For this review, take the finished solid that the model builds, in its own axes (mm). A direction names the side the tool comes from. Round coordinates to 2 decimals unless told otherwise and drop trailing zeros. Write each loop counter-clockwise with the first axis right and the second up, starting at its lowest first coordinate (ties: lowest second). Pieces come first, ordered by that corner, then holes. Notation, with made-up numbers: M 69,62.25 L 126,62.25 A19 cw 126,96.25 Z; hole C 50,52 d6. An arc over 180 degrees is marked long. Use one line per item in the form item = value. Start each with the question number.
Item 1: For faces 1 (the cylindrical face through (250.72, 2.12, 126.67)), 2 (the flat face through (284.2, 3.6, -11.4)), 3 (the cylindrical face through (270.393, 3.648, 1.982)), list the 3-axis set-ups (+Z, -Z, +X, -X, +Y, -Y) from which the entire face can be reached by the end or side of a thin tool; tool diameter is ignored.
Item 2: For line 1 (X direction, y = 1.25, z = 0.5); line 2 (Y direction, x = 275.5, z = -28); line 3 (X direction, y = 3.25, z = -28.5), list the stretches that pass through material, from the lowest coordinate up. Write a range as [from, to].
Item 3: Add section A-A (z = 92.5). State the section outline as (x, y) points.
Item 4: For P1, Ø14, axis at x = 256, z = 125, coming from the +Y side; P2, Ø1.5, axis at x = 258, z = 107, coming from the +Y side; P3, Ø3, axis at x = 257, y = 2.5, coming from the -Z side, all flat-tipped, find the tip position at first contact; note any pin that passes through.
Item 5: Draft analysis for pull direction Z (two halves, no side actions). For faces 4 (the cylindrical face through (289.992, 1.775, 2.126)), 5 (the flat face through (272, 0, 10)), 6 (the cylindrical face through (281.795, 2.121, 36.119)), state which applies: released by +Z, released by -Z, zero draft, split by the parting line, or undercut.
Item 6: Add section B-B (y = 4.75). State the section outline as (x, z) points.
Item 7: Add section C-C (z = -117). State the section outline as (x, y) points.
from build123d import *

# Parameters (mm, degrees)
AUFSATZ_LINEAR_AUSTRAGEN1_DEPTH = 3.6
SCHNITT_LINEAR_AUSTRAGEN1_DEPTH = 3
SCHNITT_LINEAR_AUSTRAGEN2_DEPTH = 325.249841943
SCHNITT_LINEAR_AUSTRAGEN3_DEPTH = 3
AUFSATZ_LINEAR_AUSTRAGEN2_DEPTH = 3.8


with BuildPart() as part:
    # Skizze1 → Aufsatz-Linear austragen1 (new body)
    with BuildSketch(Plane(origin=(0, 0, 0), x_dir=(1, 0, 0), z_dir=(0, 1, 0))):
        with BuildLine():
            Line((251.147367097, 145), (234.173269183, 135.2))
            ThreePointArc((234.173269183, 135.2), (270.4, 0), (234.173269183, -135.2))
            Line((234.173269183, -135.2), (251.147367097, -145))
            ThreePointArc((251.147367097, -145), (290, 0), (251.147367097, 145))
        make_face()
    extrude(amount=AUFSATZ_LINEAR_AUSTRAGEN1_DEPTH)

    # Skizze2 → Schnitt-Linear austragen1 (cut)
    with BuildSketch(Plane(origin=(0, 3.6, 0), x_dir=(1, 0, 0), z_dir=(0, 1, 0))):
        with BuildLine():
            Line((243.266535923, 140.45), (246.037817215, 142.05))
            ThreePointArc((246.037817215, 142.05), (284.1, 0), (246.037817215, -142.05))
            Line((246.037817215, -142.05), (243.266535923, -140.45))
            ThreePointArc((243.266535923, -140.45), (280.9, 0), (243.266535923, 140.45))
        make_face()
    extrude(amount=-SCHNITT_LINEAR_AUSTRAGEN1_DEPTH, mode=Mode.SUBTRACT)

    # Skizze3 → Schnitt-Linear austragen2 (cut, through all)
    with BuildSketch(Plane(origin=(0, 3.6, 0), x_dir=(1, 0, 0), z_dir=(0, 1, 0))):
        Polygon((276.456207793, 41.439295032), (282.404876961, 42.222452186), (283.710138883, 32.308003572), (277.761469715, 31.524846419), align=None)
        Polygon((256.310912175, -111.579417009), (261.85418937, -113.875517603), (265.681023694, -104.636722278), (260.137746499, -102.340621683), align=None)
    extrude(amount=-SCHNITT_LINEAR_AUSTRAGEN2_DEPTH, mode=Mode.SUBTRACT)

    # Skizze4 → Schnitt-Linear austragen3 (cut)
    with BuildSketch(Plane(origin=(0, 3.6, 0), x_dir=(1, 0, 0), z_dir=(0, 1, 0))):
        Polygon((256.95059542, -104.808833183), (266.189390746, -108.635667506), (265.041340448, -111.407306104), (255.802545123, -107.58047178), align=None)
        Polygon((274.930159743, 37.708185633), (284.844608357, 39.013447555), (285.236186933, 36.039112971), (275.32173832, 34.733851049), align=None)
    extrude(amount=-SCHNITT_LINEAR_AUSTRAGEN3_DEPTH, mode=Mode.SUBTRACT)

    # Skizze5 → Aufsatz-Linear austragen2 (add)
    with BuildSketch(Plane(origin=(0, 3.6, 0), x_dir=(1, 0, 0), z_dir=(0, 1, 0))):
        with BuildLine():
            Line((234.173269183, 135.2), (237.98378096, 137.4))
            ThreePointArc((237.98378096, 137.4), (274.8, 0), (237.98378096, -137.4))
            Line((237.98378096, -137.4), (234.173269183, -135.2))
            ThreePointArc((234.173269183, -135.2), (270.4, 0), (234.173269183, 135.2))
        make_face()
    extrude(amount=AUFSATZ_LINEAR_AUSTRAGEN2_DEPTH)


solid = part.part
Calculated:
q1.face_1 = +Y
q1.face_2 = +X, +Y
q1.face_3 = -X, +Y, -Y
q2.line_1 = [270.4, 280.9], [284.1, 290]
q2.line_2 = [0, 3.6]
q2.line_3 = [268.89, 279.45], [282.67, 288.6]
q3.outline = M 254.09,0 L 274.85,0 L 274.85,3.6 L 268.62,3.6 L 268.62,0.6 L 265.23,0.6 L 265.23,3.6 L 258.76,3.6 L 258.76,7.4 L 254.09,7.4 Z
q4.P1 = 3.6
q4.P2 = 0.6
q4.P3 = -137.19
q5.face_4 = split by the parting line
q5.face_5 = zero draft
q5.face_6 = undercut
q6.outline = M 234.17,-135.2 L 237.98,-137.4 A274.8 ccw 237.98,137.4 L 234.17,135.2 A270.4 cw Z
q7.outline = M 243.78,0 L 265.35,0 L 265.35,3.6 L 258.89,3.6 L 258.89,0.6 L 255.37,0.6 L 255.37,3.6 L 248.65,3.6 L 248.65,7.4 L 243.78,7.4 Z
